Autodesk Inventor part; units mm, degrees
ref_plane "YZ Plane" through (0, 0, 0) normal (1, 0, 0) x (0, 1, 0)
ref_plane "XZ Plane" through (0, 0, 0) normal (0, 1, 0) x (-1, 0, 0)
ref_plane "XY Plane" through (0, 0, 0) normal (0, 0, 1) x (1, 0, 0)
sketch "Sketch1" plane through (0, 0, 0) normal (0, 1, 0) x (-1, 0, 0)
  line L0 (15, 120) -> (-15, 120)
  line L1 (-15, 120) -> (-15, -120)
  line L2 (-15, -120) -> (15, -120)
  line L3 (15, -120) -> (15, 120)
  point P0 (0, 0)
  point P1 (0, 120)
  point P2 (15, 0)
  dimension "d0" = 240
  dimension "d1" = 30
extrude "Extrusion1" add sketch "Sketch1" along normal blind 15
sketch "Sketch2" plane through (0, 15, 0) normal (0, 1, 0) x (1, 0, 0)
  line L0 (-15, 120) -> (-15, -120)
  line L1 (15, 120) -> (-15, 120)
  line L2 (-15, -120) -> (-5, -120)
  line L3 (-5, -120) -> (-5, 120)
  line L4 (-5, 120) -> (-15, 120)
  line L5 (-15, 120) -> (-15, -120)
  point P0 (0, 0)
  dimension "d4" = 10
extrude "Extrusion2" add sketch "Sketch2" along normal blind 10
sketch "Sketch4" plane through (0, 15, 0) normal (0, 1, 0) x (1, 0, 0)
  line L0 (15, 120) -> (-5, 120)
  line L1 (15, -120) -> (15, 120)
  line L2 (15, -120) -> (0, -120)
  line L3 (0, -120) -> (0, -105)
  line L4 (0, -105) -> (15, -105)
  line L5 (15, -105) -> (15, -120)
  point P0 (0, 0)
  dimension "d42" = 15
  dimension "d43" = 15
extrude "Extrusion3" cut sketch "Sketch4" against normal blind 10
sketch "Sketch5" plane through (0, 5, 0) normal (0, 1, 0) x (1, 0, 0)
  line L0 (15, -120) -> (15, 120)
  line L1 (0, -105) -> (15, -105)
  line L2 (15, -120) -> (0, -105) construction
  line L3 (-15, -120) -> (15, -120)
  line L4 (0, -120) -> (15, -105) construction
  point P0 (0, 0)
  point P1 (7.5, -112.5)
  point P2 (7.5, -112.5)
hole "Hole2" at (7.5, 5, 112.5) direction (0, -1, 0) diameter 4 depth 4
mirror "Mirror1" about plane through (0, 0, 0) normal (0, 0, 1) of "Extrusion3", "Hole2"
move faces "Move1" translate (0, -5, 0) faces at (5, 0, 40)
move faces "Move3" translate (1.716, 0, 0) faces at (-15, 5, -40)
move faces "Move4" translate (-1.213, 0, 0) faces at (-5, 18.3333, 40)
move faces "Move5" translate (0, -4, 0) faces at (10, 15, 35)
sketch "Sketch6" plane through (-6.213, 25, 120) normal (1, 0, 0) x (0, 0, -1)
  point P0 (120, -25)
sketch "Sketch7" plane through (-6.213, 25, 120) normal (1, 0, 0) x (0, 0, -1)
  line L0 (0, 0) -> (240, 0)
  line L1 (225, -14) -> (240, -14)
  line L2 (0, -14) -> (0, 0)
  line L3 (0, -30) -> (0, 0)
  line L4 (240, -30) -> (240, 0)
  point P0 (120, -25)
  point P1 (218.75, -7)
  point P2 (178.75, -7)
  point P3 (166.25, -7)
  point P4 (126.25, -7)
  point P5 (113.75, -7)
  point P6 (73.75, -7)
  point P7 (61.25, -7)
  point P8 (0, -7)
  point P9 (21.25, -7)
  point P10 (7.4425, -7)
  point P11 (0, -7)
  point P12 (0, -7)
  point P13 (232.5575, -7)
  dimension "d82" = 40
  dimension "d83" = 12.5
  dimension "d84" = 40
  dimension "d85" = 12.5
  dimension "d86" = 40
  dimension "d87" = 12.5
  dimension "d91" = 7
  dimension "d93" = 40
  dimension "d99" = 14
  dimension "d100" = 21.25
  dimension "d101" = 7.4425
  dimension "d103" = 7.4425
hole "Hole3" at (-6.213, 18, 58.75) at (-6.213, 18, 46.25) at (-6.213, 18, 6.25) at (-6.213, 18, -6.25) at (-6.213, 18, -46.25) at (-6.213, 18, -58.75) at (-6.213, 18, -98.75) at (-6.213, 18, 98.75) at (-6.213, 18, -112.5575) at (-6.213, 18, 112.5575) direction (-1, 0, 0) diameter 6 end through all
sketch "Sketch8" plane through (15, 5, 120) normal (1, 0, 0) x (0, 0, -1)
  line L0 (240, -10) -> (240, 20)
  line L1 (0, -10) -> (0, 20)
  line L2 (240, -10) -> (240, 0)
  line L3 (203.8731, -5) -> (-4.7144, -5)
  line L4 (240, -5.9) -> (0, -5.9)
  line L5 (240, -4.1) -> (0, -4.1)
  line L6 (240, -4.1) -> (240, -5.9)
  line L7 (0, -4.1) -> (0, -5.9)
  point P0 (120, -5)
  point P1 (240, -5)
  point P2 (99.5794, -5)
  point P3 (240, -5)
  point P4 (0, -4.1)
  dimension "d78" = 1.8
extrude "Extrusion4" cut sketch "Sketch8" against normal blind 1.8
fillet "Fillet1" radius 2 1 edges at (-13.284, -5, 0)
fillet "Fillet2" radius 2 1 edges at (15, -5, 0)
properties part number "horizontal_Edge" material "ABS Plastic"
Input: part model. Units: mm. Frame: model coordinates. A direction names the side the tool comes from. Round coordinates to 2 decimals unless told otherwise and drop trailing zeros. Order: outer loops, then holes, each group sorted by start corner. A loop starts at its lowest first (then second) coordinate and runs counter-clockwise, first axis right, second up. Notation, with made-up numbers: (64, -19.5) - (74, -19.5) arc R21 cw to (74, 10.5) - close; hole circle Ø9 at (79.5, 74.25). An arc over 180 degrees is marked (long way). Use a Markdown table: item, result.
1. Material intervals for probe 1 along Y at (x, z) = (-8.5, 58.75); probe 2 along Y at (x, z) = (9.5, -22); probe 3 along Y at (x, z) = (3.5, 107), sorted ascending.
Evaluation:
| item | result |
|---|---|
| probe 1 | -5 to 15, 21 to 25 |
| probe 2 | -5 to 11 |
| probe 3 | -5 to 5 |
2. Access query for faces 4 (the face through (5, 11, 2)), 5 (the face through (5.7, 5, 114.1)), 6 (the face through (7, 1, -113)). Directions: +Z, -Z, +X, -X, +Y, -Y. A direction counts if a zero-diameter tool reaches every point of the face in a straight line with its end or side. Return the directions, or none.
Evaluation:
| item | result |
|---|---|
| face 4 | +Z, -Z, +X, +Y |
| face 5 | +Z, +X, +Y |
| face 6 | +Y |
3. First-contact query: pin 1 (3 mm diameter, centred on x = 7.5, y = 9, fed in from -Z); pin 2 (5 mm diameter, centred on y = 18, z = -98.75, fed in from -X); pin 3 (7 mm diameter, centred on y = 18, z = 98.75, fed in from +X); pin 4 (1.4 mm diameter, centred on x = 14.5, z = 47, fed in from +Y). Flat tips, straight axial feed; report the tip coordinate or a pass-through.
Evaluation:
| item | result |
|---|---|
| pin 1 | z = -105 |
| pin 2 | through |
| pin 3 | x = -6.21 |
| pin 4 | y = 11 |
4. Mould query, pull axis X, two halves, no side actions, for faces 1 (the face through (0, 8, 113)), 2 (the face through (8, 8, -105)), 3 (the face through (7, 1, 112)). Classes: +X half, -X half, draft (parallel to the pull), parting line (faces both ways), or undercut.
Evaluation:
| item | result |
|---|---|
| face 1 | +X half |
| face 2 | draft |
| face 3 | undercut |
5. Section C-C on z = 112.5. Return the cut outline in (x, y).
Evaluation:
| item | result |
|---|---|
| outline | (-13.28, -3) arc R2 ccw to (-11.28, -5) - (13, -5) arc R2 ccw to (15, -3) - (15, -0.9) - (13.2, -0.9) - (13.2, 0.9) - (15, 0.9) - (15, 5) - (9.5, 5) - (9.5, 1) - (5.5, 1) - (5.5, 5) - (0, 5) - (0, 11) - (-6.21, 11) - (-6.21, 15) - (-13.28, 15) - close; (-13.28, 21) - (-6.21, 21) - (-6.21, 25) - (-13.28, 25) - close |
6. Section B-B on z = -52. Return the cut outline in (x, y).
Evaluation:
| item | result |
|---|---|
| outline | (-13.28, -3) arc R2 ccw to (-11.28, -5) - (13, -5) arc R2 ccw to (15, -3) - (15, -0.9) - (13.2, -0.9) - (13.2, 0.9) - (15, 0.9) - (15, 11) - (-6.21, 11) - (-6.21, 25) - (-13.28, 25) - close |
7. Section A-A on z = -98.75. Return the cut outline in (x, y), then the cut area to 3 significant figures.
Evaluation:
| item | result |
|---|---|
| outline | (-13.28, -3) arc R2 ccw to (-11.28, -5) - (13, -5) arc R2 ccw to (15, -3) - (15, -0.9) - (13.2, -0.9) - (13.2, 0.9) - (15, 0.9) - (15, 11) - (-6.21, 11) - (-6.21, 15) - (-13.28, 15) - close; (-13.28, 21) - (-6.21, 21) - (-6.21, 25) - (-13.28, 25) - close |
| area | 504 mm^2 |
